Autodesk Inventor part; units mm, degrees
ref_plane "Arbeitsebene1" through (0, 0, 9.5) normal (0, 0, 1) x (1, 0, 0)
ref_plane "YZ Plane" through (0, 0, 0) normal (1, 0, 0) x (0, 1, 0)
ref_plane "XZ Plane" through (0, 0, 0) normal (0, 1, 0) x (-1, 0, 0)
sketch "Skizze1" plane through (0, 0, 0) normal (0, 0, 1) x (1, 0, 0)
  line L0 (0, 0) -> (49, 0)
  line L1 (49, 0) -> (49, 80)
  line L2 (49, 80) -> (0, 80)
  line L3 (0, 80) -> (0, 0)
  dimension "d0" = 49
  dimension "d1" = 80
extrude "Extrusion1" add sketch "Skizze1" along normal blind 19
sketch "Skizze2" plane through (0, 80, 0) normal (0, 1, 0) x (1, 0, 0)
  line L0 (0, 0) -> (0, -19)
  point P0 (7, -9.5)
  point P1 (0, -9.5)
  point P2 (42, -9.5)
  dimension "d11" = 7
  dimension "d12" = 35
hole "Bohrung1" at (7, 80, 9.5) at (42, 80, 9.5) direction (0, -1, 0) diameter 4.917 depth 17.1 tip angle 118
sketch "Skizze3" plane through (0, 0, 0) normal (0, -1, 0) x (1, 0, 0)
  line L0 (0, 0) -> (0, 19)
  point P0 (9.5, 9.5)
  point P1 (0, 9.5)
  point P2 (0, 9.5)
  point P3 (0, 9.5)
  point P4 (39.5, 9.5)
  dimension "d20" = 9.5
  dimension "d21" = 30
hole "Bohrung2" at (9.5, 0, 9.5) at (39.5, 0, 9.5) direction (0, 1, 0) diameter 6.647 depth 22.2 tip angle 118
ref_plane "Arbeitsebene1" through (0, 0, 9.5) normal (0, 0, 1) x (1, 0, 0)
sketch "Skizze6" plane through (0, 0, 9.5) normal (0, 0, 1) x (1, 0, 0)
  line L0 (49, 0) -> (49, 80)
  line L1 (49, 80) -> (0, 80)
  point P0 (0, 0)
  point P1 (24.5, 40)
  point P2 (49, 40)
  point P3 (24.5, 80)
hole "Bohrung4" at (24.5, 40, 9.5) direction (0, 0, 1) diameter 35 end through all counterbore diameter 36 counterbore depth 2
hole "Bohrung5" at (24.5, 40, 9.5) direction (0, 0, -1) diameter 30 end through all
properties part number "Lagerbock" material "Stahl, galvanisiert"
The listing builds one solid part. Answer for the finished solid, in the listing's coordinates (mm). A direction names the side the tool comes from. Coordinates: 2 decimals unless noted, no trailing zeros. Order: outer loops, then holes, each group sorted by start corner. A loop starts at its lowest first (then second) coordinate and runs counter-clockwise, first axis right, second up.
Q1. A cutting plane is placed at A-A, the plane y = 6. Write down the section's boundary in (x, z).
Q2. For a pull along X with two mould halves and no side action, classify faces 1 (the face through (0, 41, 9)), 2 (the face through (24, 58, 19)), 3 (the face through (38.99, 23.85, 9.23)) as pulls with the +X half, pulls with the -X half, needs draft (parallel to the pull), parting line crosses it, or undercut.
Q3. Consider line 1 (X direction, y = 69.75, z = 9.5); line 2 (X direction, y = 16, z = 9.5); line 3 (X direction, y = 40, z = 10.6). Determine where each line is inside the solid, lowest interval first.
Q4. A cutting plane is placed at C-C, the plane z = 4.75. Write down the section's boundary in (x, y), and give its area (3 significant figures).
Q5. A cutting plane is placed at D-D, the plane y = 41. Write down the section's boundary in (x, z), and give its area (3 significant figures).
Q6. Which of the six approach directions +Z, -Z, +X, -X, +Y, -Y give full straight-line access (tool end or side, diameter ignored) to faces 4 (the face through (31.39, 56.63, 10.51)), 5 (the face through (43.5, 71.33, 7.55)), 6 (the face through (25, 80, 9)), 7 (the face through (40.77, 11.26, 6.43)), 8 (the face through (49, 39, 9))?
Q7. A cutting plane is placed at B-B, the plane x = 20.5. Write down the section's boundary in (y, z).
Q8. Given P1, Ø4, axis at x = 36.5, y = 11.5, coming from the -Z side; P2, Ø21, axis at x = 24.5, y = 40, coming from the +Z side; P3, Ø1, axis at x = 11.5, z = 11, coming from the -Y side, each flat-ended and moving along its own axis, determine where each tip first touches the part or whether it passes through.
Answers follow:
1. outline: (0, 0) - (49, 0) - (49, 19) - (0, 19) - close; hole circle Ø6.65 at (9.5, 9.5); hole circle Ø6.65 at (39.5, 9.5)
2. face 1: pulls with the -X half
2. face 2: needs draft
2. face 3: undercut
3. line 1: x = 0 to 4.54, 9.46 to 39.54, 44.46 to 49
3. line 2: x = 0 to 6.18, 12.82 to 36.18, 42.82 to 49
3. line 3: x = 0 to 6.5, 42.5 to 49
4. outline: (0, 0) - (49, 0) - (49, 80) - (0, 80) - close; hole circle Ø30 at (24.5, 40)
4. area: 3,210 mm2
5. outline: (0, 0) - (9.53, 0) - (9.53, 9.5) - (6.53, 9.5) - (6.53, 11.5) - (7.03, 11.5) - (7.03, 19) - (0, 19) - close; (39.47, 0) - (49, 0) - (49, 19) - (41.97, 19) - (41.97, 11.5) - (42.47, 11.5) - (42.47, 9.5) - (39.47, 9.5) - close
5. area: 313 mm2
6. face 4: none
6. face 5: +Y
6. face 6: +Z, -Z, +X, -X, +Y
6. face 7: -Y
6. face 8: +Z, -Z, +X, +Y, -Y
7. outline: (0, 0) - (25.54, 0) - (25.54, 9.5) - (22.45, 9.5) - (22.45, 11.5) - (22.96, 11.5) - (22.96, 19) - (0, 19) - close; (54.46, 0) - (80, 0) - (80, 19) - (57.04, 19) - (57.04, 11.5) - (57.55, 11.5) - (57.55, 9.5) - (54.46, 9.5) - close
8. P1: stops at z = 0
8. P2: passes through
8. P3: stops at y = 22.39
